Autodesk Inventor part; units mm, degrees
ref_plane "YZ Plane" through (0, 0, 0) normal (1, 0, 0) x (0, 1, 0)
ref_plane "XZ Plane" through (0, 0, 0) normal (0, 1, 0) x (-1, 0, 0)
ref_plane "XY Plane" through (0, 0, 0) normal (0, 0, 1) x (1, 0, 0)
sketch "Base" plane through (0, 0, 0) normal (0, 0, 1) x (1, 0, 0)
  line L0 (-27, -40) -> (27, -40)
  line L1 (27, -40) -> (27, 40)
  line L2 (27, 40) -> (-27, 40)
  line L3 (-27, 40) -> (-27, -40)
  line L4 (-27, -40) -> (27, 40) construction
  line L5 (27, -40) -> (-27, 40) construction
  point P0 (0, 0)
  dimension "d0" = 80
  dimension "d1" = 54
extrude "BaseFeature" add sketch "Base" along normal blind 48
sketch "DINRail" plane through (-27, -40, 0) normal (-1, 0, 0) x (0, 0, 1)
  line L0 (0, 80) -> (0, 0) construction
  line L1 (0, 0) -> (48, 0) construction
  line L2 (48, 80) -> (48, 0) construction
  line L3 (0, 80) -> (48, 80) construction
  line L4 (0, 57.7) -> (4, 57.7)
  line L5 (4, 57.7) -> (4, 22.3)
  line L6 (4, 22.3) -> (0, 22.3)
  line L7 (0, 22.3) -> (0, 57.7)
  line L8 (0, 57.7) -> (4, 22.3) construction
  line L9 (4, 57.7) -> (0, 22.3) construction
  line L10 (0, -16) -> (0, 96)
  line L11 (-9.6, 40) -> (57.6, 40) construction
  line L12 (0, 80) -> (0, 0)
  point P0 (2, 40)
  point P1 (0, -16)
  point P2 (0, 96)
  dimension "d4" = 4
  dimension "d5" = 35.4
extrude "DinRailFeature" cut sketch "DINRail" against normal through all
sketch "Chamfers" plane through (-27, -40, 48) normal (-1, 0, 0) x (0, 0, 1)
  line L0 (-44, 22.3) -> (-48, 22.3) construction
  line L1 (-48, 22.3) -> (-48, 0) construction
  line L2 (-48, 0) -> (0, 0)
  line L3 (0, 80) -> (0, 0)
  line L4 (-48, 80) -> (0, 80)
  line L5 (-48, 80) -> (-48, 57.7) construction
  line L6 (-48, 57.7) -> (-44, 57.7) construction
  line L7 (-44, 57.7) -> (-44, 22.3) construction
  line L8 (-3.6, 80) -> (0, 74)
  line L9 (-57.6, 40) -> (9.6, 40) construction
  line L10 (-3.6, 0) -> (0, 6)
  point P0 (-48, 40)
  point P1 (0, 6)
  point P2 (-3.6, 0)
  dimension "d8" = 6
  dimension "d9" = 3.6
extrude "ChamfersFeature" cut sketch "Chamfers" against normal through all
sketch "Screen" plane through (0, 0, 48) normal (0, 0, 1) x (1, 0, 0)
  line L0 (27, -34) -> (27, 34)
  line L1 (-27, 22.5) -> (27, 22.5)
  line L2 (27, 22.5) -> (27, -22.5)
  line L3 (27, -22.5) -> (-27, -22.5)
  line L4 (-27, -22.5) -> (-27, 22.5)
  line L5 (-27, 22.5) -> (27, -22.5) construction
  line L6 (27, 22.5) -> (-27, -22.5) construction
  point P0 (0, 0)
  dimension "d12" = 45
extrude "ScreenFeature" add sketch "Screen" along normal blind 16
sketch "ScreenBezel" plane through (0, 0, 64) normal (0, 0, 1) x (1, 0, 0)
  line L0 (-24.5, -20) -> (24.5, -20)
  line L1 (24.5, -20) -> (24.5, 20)
  line L2 (24.5, 20) -> (-24.5, 20)
  line L3 (-24.5, 20) -> (-24.5, -20)
  line L4 (-24.5, -20) -> (24.5, 20) construction
  line L5 (24.5, -20) -> (-24.5, 20) construction
  line L6 (27, 22.5) -> (-27, 22.5)
  line L7 (27, -22.5) -> (27, 22.5)
  point P0 (0, 0)
  dimension "d15" = 2.5
  dimension "d16" = 2.5
extrude "ScreenBezelFeature" cut sketch "ScreenBezel" against normal blind 1
chamfer "ScreenChamferFeature" distance 1 angle 45 4 edges at (-24.5, 0, 63) (0, 20, 63) (24.5, 0, 63) (0, -20, 63)
sketch "SupplyTerminals" plane through (0, 0, 48) normal (0, 0, 1) x (1, 0, 0)
  line L0 (-27, -40) -> (27, -40)
  line L1 (-27, -34) -> (27, -34)
  line L2 (-22, -40) -> (-16, -40)
  line L3 (-16, -40) -> (-16, -34)
  line L4 (-16, -34) -> (-22, -34)
  line L5 (-22, -34) -> (-22, -40)
  circle A0 centre (-19, -34) radius 3
  line L6 (-27, -40) -> (-27, -34)
  line L7 (27, -22.5) -> (-27, -22.5)
  line L8 (-14, -22.5) -> (-14, -40) construction
  line L9 (-6, -40) -> (-12, -40)
  line L10 (-12, -40) -> (-12, -34)
  line L11 (-6, -34) -> (-6, -40)
  circle A1 centre (-9, -34) radius 3
  point P0 (0, 0)
  dimension "d23" = 6
  dimension "d24" = 5
  dimension "d25" = 2
extrude "SupplyTerminalsFeature" cut sketch "SupplyTerminals" against normal up to surface (3.6 mm away) contours L5 A0 L3 L0 | A0 L1 | L1 A0 | L10 A1 L11 L0 | A1 L1 | L1 A1
sketch "TerminalScrews" plane through (-19, -34, 44.4) normal (0, 0, 1) x (1, 0, 0)
  arc A0 (3, 0) -> (-3, 0) centre (0, 0) ccw
  arc A1 (13, 0) -> (7, 0) centre (10, 0) ccw
  circle A2 centre (0, 0) radius 2.5
  circle A3 centre (10, 0) radius 2.5
  point P0 (19, 34)
  dimension "d28" = 5
extrude "TerminalScrewsFeature" cut sketch "TerminalScrews" against normal blind 1
properties part number "EnergyMeter"
The model under review builds one solid part; all positions refer to its coordinate system, in mm. A direction names the side the tool comes from. Round coordinates to 2 decimals unless told otherwise and drop trailing zeros. Loops run counter-clockwise (first coordinate to the right, second up) from the corner with the lowest first, then second, coordinate; pieces in that order, holes last. Notation, with made-up numbers: (85, 38.5) -> (114, 38.5) arc R19 ccw to (114, 43.5) -> close; hole circle Ø1 at (35.5, -28.75). An arc over 180 degrees is marked (long way). Answer as a JSON object with one key per item and string values. Group by question number.
1) For line 1 (Y direction, x = -9, z = 44); line 2 (Y direction, x = -9, z = 3); line 3 (Y direction, x = 10.5, z = 49.5), list the stretches that pass through material, from the lowest coordinate up. Write a range as [from, to].
2) For faces 1 (the face through (0, 28, 48)), 2 (the face through (0, 17.7, 2)), 3 (the face through (-22, -36, 45)), 4 (the face through (-19, -34, 43.4)), list the 3-axis set-ups (+Z, -Z, +X, -X, +Y, -Y) from which the entire face can be reached by the end or side of a thin tool; tool diameter is ignored.
3) For pin 1 Ø6 at (x, y) = (11, 27.5) entering from +Z; pin 2 Ø2.5 at (x, y) = (-19, -33) entering from +Z; pin 3 Ø4 at (x, y) = (-8.5, -35) entering from +Z, all flat-tipped, find the tip position at first contact; note any pin that passes through.
4) We need section C-C on z = 51. Write out the cut boundary in (x, y), then the cut area to 3 significant figures.
Result set:
{
 "1": {"line 1": "[-40, -36.5], [-31.5, 40]", "line 2": "[-40, -17.7], [17.7, 40]", "line 3": "[-22.5, 22.5]"},
 "2": {"face 1": "+Z, +X, -X, +Y", "face 2": "-Z, +X, -X", "face 3": "+Z, -Y", "face 4": "+Z"},
 "3": {"pin 1": "z = 48", "pin 2": "z = 43.4", "pin 3": "z = 44.4"},
 "4": {"outline": "(-27, -22.5) -> (27, -22.5) -> (27, 22.5) -> (-27, 22.5) -> close", "area": "2,430 mm²"}
}
